Design review of the part built by this model. Coordinates are the model's own, in mm. Face numbers are marked on the shaded views. A direction names the side the tool comes from. Coordinates: 2 decimals unless noted, no trailing zeros. Write each loop counter-clockwise with the first axis right and the second up, starting at its lowest first coordinate (ties: lowest second). Pieces come first, ordered by that corner, then holes.
```python
from build123d import *

# Parameters (mm, degrees)
SKETCH1_R           = 75
BOSS_EXTRUDE1_DEPTH = 10
CUT_EXTRUDE1_REACH  = 12
SKETCH2_R           = 3
SKETCH3_W           = 60
SKETCH3_H           = 10
BOSS_EXTRUDE2_DEPTH = 60
SKETCH4_R           = 9
CUT_EXTRUDE2_DEPTH  = 101
SKETCH6_R           = 9
SKETCH6_R_2         = 4.5
BOSS_EXTRUDE3_DEPTH = 4
SKETCH9_R           = 2.25
CUT_EXTRUDE5_DEPTH  = 10


with BuildPart() as part:
    # Sketch1 → Boss-Extrude1 (new body)
    with BuildSketch(Plane.XY):
        Circle(SKETCH1_R)
    extrude(amount=BOSS_EXTRUDE1_DEPTH)

    # Sketch2 → Cut-Extrude1 (cut, up to next)
    with BuildSketch(Plane.XY.offset(10), mode=Mode.PRIVATE) as cut_extrude1_sk1:
        Circle(SKETCH2_R)
    cut_extrude1_tool1 = extrude(cut_extrude1_sk1.sketch, amount=-CUT_EXTRUDE1_REACH, mode=Mode.PRIVATE) & part.part
    add(cut_extrude1_tool1.solids().sort_by_distance((0, 0, 10))[0], mode=Mode.SUBTRACT)

    # Sketch3 → Boss-Extrude2 (add)
    with BuildSketch(Plane(origin=(0, 0, 0), x_dir=(-1, 0, 0), z_dir=(0, 0, -1))):
        with Locations((0, 20)):
            Rectangle(SKETCH3_W, SKETCH3_H)
        with Locations((0, -20)):
            Rectangle(SKETCH3_W, SKETCH3_H)
    extrude(amount=BOSS_EXTRUDE2_DEPTH)

    # Sketch4 → Cut-Extrude2 (cut, through all)
    with BuildSketch(Plane.XZ.offset(25)):
        with Locations((0, -37.6)):
            Circle(SKETCH4_R)
    extrude(amount=-CUT_EXTRUDE2_DEPTH, mode=Mode.SUBTRACT)

    # Sketch6 → Boss-Extrude3 (add)
    with BuildSketch(Plane.XZ.offset(-15)):
        with Locations((0, -37.6)):
            Circle(SKETCH6_R)
        with Locations((0, -37.6)):
            Circle(SKETCH6_R_2, mode=Mode.SUBTRACT)
    boss_extrude3 = extrude(amount=-BOSS_EXTRUDE3_DEPTH)

    # Sketch9 → Cut-Extrude5 (cut)
    with BuildSketch(Plane.XZ.offset(25)):
        with Locations((-5, -2.5)):
            Circle(SKETCH9_R)
        with Locations((5, -2.5)):
            Circle(SKETCH9_R)
        with Locations((-5, -53)):
            Circle(SKETCH9_R)
        with Locations((5.285793913, -53)):
            Circle(SKETCH9_R)
    extrude(amount=-CUT_EXTRUDE5_DEPTH, mode=Mode.SUBTRACT)

    # Mirror1: Boss-Extrude3 across plane
    add(boss_extrude3.mirror(Plane.ZX))


solid = part.part
```
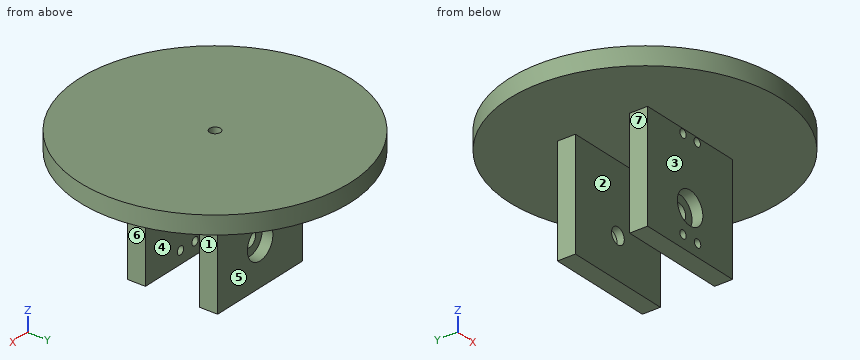
(1) Consider section C-C (z = -21). Give the boundary of the cut face in (x, y), plus the area to 3 significant figures.
(2) For the marked faces 5, 6 and 7, list the 3-axis set-ups (+Z, -Z, +X, -X, +Y, -Y) from which the entire face can be reached by the end or side of a thin tool; tool diameter is ignored.
(3) Consider section B-B (z = -2.5). Give the boundary of the cut face in (x, y), plus the area to 3 significant figures.
(4) Consider section A-A (y = 0). Give the boundary of the cut face in (x, z).
(5) Consider section D-D (x = 17.5). Give the boundary of the cut face in (y, z), plus the area to 3 significant figures.
(6) Mouldability with a two-part tool opening along Y and no side actions: class the marked faces 1, 2, 3 and 4 as +Y half, -Y half, draft (parallel to the pull), parting line (faces both ways), or undercut.
(7) Wall thickness on line 1 (Z direction, x = 0, y = 17.25); line 2 (Z direction, x = -5, y = -20.5); line 3 (Y direction, x = 29, z = -9): over which ranges is each line inside the solid? List them lowest first.
(8) Insertion check: pin 1 Ø6 at (x, z) = (5, -2.5) entering from -Y; pin 2 Ø12 at (x, y) = (30.5, 43.5) entering from -Z; pin 3 Ø1 at (x, z) = (-8, -6.5) entering from +Y. Each pin has a flat end and moves straight along its axis. Give the tip position at first contact, or say it passes through.
Results:
1. outline: (-30, -25) - (30, -25) - (30, -15) - (-30, -15) - close; (-30, 15) - (30, 15) - (30, 25) - (-30, 25) - close
1. area: 1,200 mm2
2. face 5: -Z, +X, -X, +Y
2. face 6: -Z, +X, +Y, -Y
2. face 7: -Z, -X, +Y, -Y
3. outline: (-30, -25) - (-7.25, -25) - (-7.25, -15) - (-30, -15) - close; (-30, 15) - (30, 15) - (30, 25) - (-30, 25) - close; (-2.75, -25) - (2.75, -25) - (2.75, -15) - (-2.75, -15) - close; (7.25, -25) - (30, -25) - (30, -15) - (7.25, -15) - close
3. area: 1,110 mm2
4. outline: (-75, 0) - (-3, 0) - (-3, 10) - (-75, 10) - close; (3, 0) - (75, 0) - (75, 10) - (3, 10) - close
5. outline: (-72.93, 0) - (-25, 0) - (-25, -60) - (-15, -60) - (-15, 0) - (15, 0) - (15, -60) - (25, -60) - (25, 0) - (72.93, 0) - (72.93, 10) - (-72.93, 10) - close
5. area: 2,660 mm2
6. face 1: draft
6. face 2: undercut
6. face 3: -Y half
6. face 4: undercut
7. line 1: z = -60 to -42.1, -33.1 to 10
7. line 2: z = -60 to -55.25, -50.75 to -45.08, -30.12 to -4.75, -0.25 to 10
7. line 3: y = -25 to -15, 15 to 25
8. pin 1: stops at y = -74.93
8. pin 2: stops at z = 0
8. pin 3: stops at y = 25
